Verification items for the finished model (mm, model axes). A direction names the side the tool comes from. Round coordinates to 2 decimals unless told otherwise and drop trailing zeros. Order: outer loops, then holes, each group sorted by start corner. A loop starts at its lowest first (then second) coordinate and runs counter-clockwise, first axis right, second up. Notation, with made-up numbers: M 34,0.5 L 47,0.5 A25 ccw 47,39.5 Z; hole C 69,-23.5 d1. An arc over 180 degrees is marked long. Answer as a JSON object with one key per item and string values. Group by question number.
```python
from build123d import *

# Parameters (mm, degrees)
SKETCH1_R           = 3.175
BOSS_EXTRUDE1_DEPTH = 4.7625
SKETCH2_R           = 3.175
SKETCH2_R_2         = 1.5875
CUT_EXTRUDE1_DEPTH  = 3.175
SKETCH3_R           = 0.396875
CUT_EXTRUDE2_DEPTH  = 5.7625


with BuildPart() as part:
    # Sketch1 → Boss-Extrude1 (new body)
    with BuildSketch(Plane(origin=(0, 0, 0), x_dir=(1, 0, 0), z_dir=(0, 1, 0))):
        Circle(SKETCH1_R)
    extrude(amount=BOSS_EXTRUDE1_DEPTH)

    # Sketch2 → Cut-Extrude1 (cut)
    with BuildSketch(Plane(origin=(0, 4.7625, 0), x_dir=(1, 0, 0), z_dir=(0, 1, 0))):
        Circle(SKETCH2_R)
        Circle(SKETCH2_R_2, mode=Mode.SUBTRACT)
    extrude(amount=-CUT_EXTRUDE1_DEPTH, mode=Mode.SUBTRACT)

    # Sketch3 → Cut-Extrude2 (cut, through all)
    with BuildSketch(Plane(origin=(0, 4.7625, 0), x_dir=(1, 0, 0), z_dir=(0, 1, 0))):
        Circle(SKETCH3_R)
    extrude(amount=-CUT_EXTRUDE2_DEPTH, mode=Mode.SUBTRACT)

    # Sketch4 → Cut-Revolve1 (revolve, cut)
    with BuildSketch(Plane(origin=(0, 0, 0), x_dir=(0, 0, -1), z_dir=(1, 0, 0))):
        Polygon((0, 0), (0, 0.79375), (-0.79375, 0), align=None)
    revolve(axis=Axis((0, 0, 0), (0, 1, 0)), mode=Mode.SUBTRACT)


solid = part.part
```
Q1. Cross-section at C-C, the plane y = 1.5. Record the cut outline in (x, z) (3 decimals).
Q2. Tool access check on faces 1 (the face through (1.4, 1.588, 1.4)), 2 (the face through (1, 0, 1)). Record the directions out of +Z, -Z, +X, -X, +Y, -Y that give a thin tool (end or side, any length) a straight path to the whole face; none if there is none.
Q3. Cross-section at B-B, the plane z = 0. Record the cut outline in (x, y) (1 decimal).
Q4. Cross-section at A-A, the plane x = 0. Record the cut outline in (y, z) (1 decimal), then the cut area to 3 significant figures.
Q5. Cross-section at D-D, the plane z = 1.25. Record the cut outline in (x, y).
Q6. Gauge pin test, flat end, axial feed: pin 1 Ø1 at (y, z) = (4.5, 1.5) entering from -X. Record the tip position at first contact, or that the pin passes through.
Q7. Thickness scan on line 1 (Z direction, x = 0, y = 3.3); line 2 (X direction, y = 1.4, z = 0) (3 decimals). Record the ranges inside material, lowest first. Write a range as from..to.
Conclusion:
{
 "1": {"outline": "C 0,0 d6.35; hole C 0,0 d0.794"},
 "2": {"face 1": "+Y", "face 2": "+Z, -Z, +X, -X, -Y"},
 "3": {"outline": "M -3.2,0 L -0.8,0 L -0.4,0.4 L -0.4,4.8 L -1.6,4.8 L -1.6,1.6 L -3.2,1.6 Z; M 0.4,0.4 L 0.8,0 L 3.2,0 L 3.2,1.6 L 1.6,1.6 L 1.6,4.8 L 0.4,4.8 Z"},
 "4": {"outline": "M 0,-3.2 L 1.6,-3.2 L 1.6,-1.6 L 4.8,-1.6 L 4.8,-0.4 L 0.4,-0.4 L 0,-0.8 Z; M 0,0.8 L 0.4,0.4 L 4.8,0.4 L 4.8,1.6 L 1.6,1.6 L 1.6,3.2 L 0,3.2 Z", "area": "16.2 mm2"},
 "5": {"outline": "M -2.92,0 L 2.92,0 L 2.92,1.59 L 0.98,1.59 L 0.98,4.76 L -0.98,4.76 L -0.98,1.59 L -2.92,1.59 Z"},
 "6": {"pin 1": "x = -1.23"},
 "7": {"line 1": "-1.59..-0.4, 0.4..1.59", "line 2": "-3.175..-0.397, 0.397..3.175"}
}
